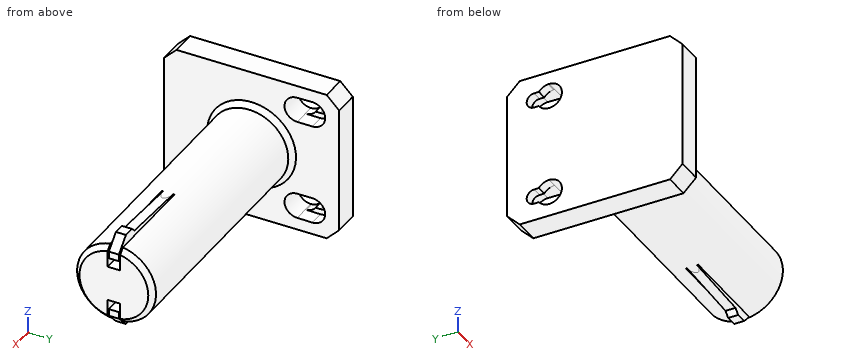
from build123d import *

# Parameters (mm, degrees)
SKETCH1_W            = 60.5
SKETCH1_H            = 70
BOSS_EXTRUDE1_DEPTH  = 10
SKETCH2_R            = 15.75
BOSS_EXTRUDE2_DEPTH  = 101.6
CUT_EXTRUDE1_DEPTH   = 40
SKETCH8_W            = 3.25
SKETCH8_H            = 5
CUT_EXTRUDE2_DEPTH   = 40
CHAMFER3_SIZE        = 2
BOSS_EXTRUDE9_DEPTH  = 4
BOSS_EXTRUDE10_DEPTH = 4
CHAMFER4_SIZE        = 5
CUT_EXTRUDE9_DEPTH   = 4
CHAMFER6_SIZE        = 2


with BuildPart() as part:
    # Sketch1 → Boss-Extrude1 (new body)
    with BuildSketch(Plane(origin=(0, 0, 0), x_dir=(0, 0, -1), z_dir=(1, 0, 0))):
        with Locations((0.23118778, -0.809157231)):
            Rectangle(SKETCH1_W, SKETCH1_H)
        with BuildLine():
            Line((-14.90655725, 23.440204594), (-14.924987971, 17.440316828))
            ThreePointArc((-14.924987971, 17.440316828), (-20.01881222, 12.34649258), (-25.112636468, 17.440316828))
            Line((-25.112636468, 17.440316828), (-25.204464795, 23.440204594))
            ThreePointArc((-25.204464795, 23.440204594), (-20.055511023, 28.589158366), (-14.90655725, 23.440204594))
        make_face(mode=Mode.SUBTRACT)
        with BuildLine():
            ThreePointArc((15.368932811, 23.440204594), (20.517886583, 28.589158366), (25.666840355, 23.440204594))
            Line((25.666840355, 23.440204594), (25.575012029, 17.440316828))
            ThreePointArc((25.575012029, 17.440316828), (20.48118778, 12.34649258), (15.387363532, 17.440316828))
            Line((15.387363532, 17.440316828), (15.368932811, 23.440204594))
        make_face(mode=Mode.SUBTRACT)
    extrude(amount=BOSS_EXTRUDE1_DEPTH)

    # Sketch2 → Boss-Extrude2 (add)
    with BuildSketch(Plane(origin=(10, 0, 0), x_dir=(0, 0, -1), z_dir=(1, 0, 0))):
        with Locations((0.23118778, -0.809157231)):
            Circle(SKETCH2_R)
    extrude(amount=BOSS_EXTRUDE2_DEPTH)

    # Sketch3 → Cut-Extrude1 (cut)
    with BuildSketch(Plane(origin=(111.6, 0, 0), x_dir=(0, 0, -1), z_dir=(1, 0, 0))):
        Polygon((-15.51881222, 1.190842769), (-10.51881222, 1.190842769), (-10.51881222, -2.809157231), (-15.51881222, -2.809157231), (-15.51881222, -3.309157231), (-10.01881222, -3.309157231), (-10.01881222, 1.690842769), (-15.51881222, 1.690842769), align=None)
        Polygon((15.98118778, -2.809157231), (15.98118778, -3.309157231), (10.48118778, -3.309157231), (10.48118778, 1.690842769), (15.98118778, 1.690842769), (15.98118778, 1.190842769), (10.98118778, 1.190842769), (10.98118778, -2.809157231), align=None)
    extrude(amount=-CUT_EXTRUDE1_DEPTH, mode=Mode.SUBTRACT)

    # Sketch8 → Cut-Extrude2 (cut)
    with BuildSketch(Plane(origin=(111.6, 0, 0), x_dir=(0, 0, -1), z_dir=(1, 0, 0))):
        with Locations((8.85618778, -0.809157231)):
            Rectangle(SKETCH8_W, SKETCH8_H)
        with Locations((-8.39381222, -0.809157231)):
            Rectangle(SKETCH8_W, SKETCH8_H)
    extrude(amount=-CUT_EXTRUDE2_DEPTH, mode=Mode.SUBTRACT)

    # Chamfer3
    chamfer3_edges = [part.edges().sort_by_distance(p)[0] for p in [
        (111.6, -16.559157231, -0.23118778),
        (111.6, 14.940842769, -0.23118778),
    ]]
    chamfer(chamfer3_edges, length=CHAMFER3_SIZE)

    # Sketch19 → Boss-Extrude9 (add)
    with BuildSketch(Plane.ZY):
        with BuildLine():
            Line((-25.666840355, 23.440204594), (-25.575012029, 17.440316828))
            ThreePointArc((-25.575012029, 17.440316828), (-25.569608823, 17.67487337), (-25.553410667, 17.908932306))
            ThreePointArc((-25.553410667, 17.908932306), (-24.917258091, 19.94397928), (-23.503874553, 21.540366846))
            Line((-23.503874553, 21.540366846), (-23.503874553, 23.440204594))
            ThreePointArc((-23.503874553, 23.440204594), (-20.517886583, 26.426192563), (-17.531898613, 23.440204594))
            Line((-17.531898613, 23.440204594), (-17.531898613, 21.593476936))
            ThreePointArc((-17.531898613, 21.593476936), (-15.9551406, 19.777396716), (-15.387363532, 17.440316828))
            Line((-15.387363532, 17.440316828), (-15.368932811, 23.440204594))
            ThreePointArc((-15.368932811, 23.440204594), (-20.517886583, 28.589158366), (-25.666840355, 23.440204594))
        make_face()
        with BuildLine():
            ThreePointArc((25.204464795, 23.440204594), (20.055511023, 28.589158366), (14.90655725, 23.440204594))
            Line((14.90655725, 23.440204594), (14.924987971, 17.440316828))
            ThreePointArc((14.924987971, 17.440316828), (15.49276504, 19.777396716), (17.069523053, 21.593476936))
            Line((17.069523053, 21.593476936), (17.069523053, 23.440204594))
            ThreePointArc((17.069523053, 23.440204594), (20.055511023, 26.426192563), (23.041498992, 23.440204594))
            Line((23.041498992, 23.440204594), (23.041498992, 21.540366846))
            ThreePointArc((23.041498992, 21.540366846), (24.454882531, 19.94397928), (25.091035106, 17.908932306))
            ThreePointArc((25.091035106, 17.908932306), (25.107233262, 17.67487337), (25.112636468, 17.440316828))
            Line((25.112636468, 17.440316828), (25.204464795, 23.440204594))
        make_face()
    extrude(amount=-BOSS_EXTRUDE9_DEPTH)

    # Sketch23 → Boss-Extrude10 (add)
    with BuildSketch(Plane(origin=(0, 1.190842769, 0), x_dir=(1, 0, 0), z_dir=(0, 1, 0))):
        Polygon((71.6, 15.78150932), (100.084633461, 17.181034874), (102.038578597, 19.029077367), (111.6, 19.029077367), (111.6, 15.78150932), align=None)
        Polygon((100.084633461, -16.718659314), (102.038578597, -18.566701807), (111.6, -18.566701807), (111.6, -15.31913376), (71.6, -15.31913376), align=None)
    extrude(amount=-BOSS_EXTRUDE10_DEPTH)

    # Chamfer4
    chamfer4_edges = [part.edges().sort_by_distance(p)[0] for p in [
        (5, -35.809157231, 30.01881222),
        (5, 34.190842769, 30.01881222),
        (5, 34.190842769, -30.48118778),
        (5, -35.809157231, -30.48118778),
    ]]
    chamfer(chamfer4_edges, length=CHAMFER4_SIZE)

    # Sketch28 → Cut-Extrude9 (cut)
    with BuildSketch(Plane(origin=(0, 1.190842769, 0), x_dir=(1, 0, 0), z_dir=(0, 1, 0))):
        Polygon((111.6, 13.752005063), (105.070544586, 20.392137095), (111.6, 20.392137095), align=None)
        Polygon((111.6, -19.929761535), (111.6, -13.289629503), (105.070544586, -19.929761535), align=None)
    extrude(amount=-CUT_EXTRUDE9_DEPTH, mode=Mode.SUBTRACT)

    # Chamfer6
    chamfer6_edges = [part.edges().sort_by_distance(p)[0] for p in [
        (10, -0.809157231, 15.51881222),
    ]]
    chamfer(chamfer6_edges, length=CHAMFER6_SIZE)


solid = part.part
The model under review builds one solid part; all positions refer to its coordinate system, in mm. Coordinates: 2 decimals unless noted, no trailing zeros. Loops run counter-clockwise (first coordinate to the right, second up) from the corner with the lowest first, then second, coordinate; pieces in that order, holes last.
(1) Consider section A-A, the plane y = 20. Give the boundary of the cut face in (x, z), plus the area to 3 significant figures.
Determined:
outline: (0, -30.48) - (10, -30.48) - (10, -25.61) - (4, -25.61) - (4, -24.89) - (0, -24.89) - close; (0, -16.08) - (4, -16.08) - (4, -15.38) - (10, -15.38) - (10, 14.92) - (4, 14.92) - (4, 15.61) - (0, 15.61) - close; (0, 24.42) - (4, 24.42) - (4, 25.15) - (10, 25.15) - (10, 30.02) - (0, 30.02) - close
area: 412 mm2
(2) Insertion check: P1, Ø7, axis at x = 99, z = -13.5, coming from the -Y side; P2, Ø8, axis at x = 25.5, z = 11.5, coming from the -Y side; P3, Ø3, axis at y = 20.5, z = 20.5, coming from the +X side; P4, Ø11.5, axis at y = 21, z = -22, coming from the +X side. Each pin has a flat end and moves straight along its axis. Give the tip position at first contact, or say it passes through.
Determined:
P1: stops at y = -13.16
P2: stops at y = -14.53
P3: passes through
P4: stops at x = 10
(3) Consider section B-B, the plane x = 81. Give the boundary of the cut face in (y, z).
Determined:
outline: (-3.31, -15.78) - (-3.31, -7.23) - (1.69, -7.23) - (1.69, -15.78) arc R15.75 ccw to (1.69, 15.32) - (1.69, 6.77) - (-3.31, 6.77) - (-3.31, 15.32) arc R15.75 ccw to start; (-2.81, -16.24) - (1.19, -16.24) - (1.19, -10.98) - (-2.81, -10.98) - close; (-2.81, 10.52) - (1.19, 10.52) - (1.19, 15.78) - (-2.81, 15.78) - close
(4) Consider section C-C, the plane z = 21. Give the boundary of the cut face in (x, y), plus the area to 3 significant figures.
Determined:
outline: (0, -35.81) - (10, -35.81) - (10, 12.44) - (0, 12.44) - close; (0, 26.27) - (4, 26.27) - (4, 28.5) - (10, 28.5) - (10, 34.19) - (0, 34.19) - close
area: 548 mm2
(5) Wall thickness on L1, parallel to X at y = 22, z = -25; L2, parallel to X at y = -29.5, z = 27.5; L3, parallel to Z at x = 41.5, y = -0.5: over which ranges is each line inside the solid? List them lowest first.
Determined:
L1: x = 0 to 4
L2: x = 0 to 10
L3: z = -15.98 to 15.52
(6) Consider section D-D, the plane y = -23. Give the boundary of the cut face in (x, z), plus the area to 3 significant figures.
Determined:
outline: (0, -30.48) - (10, -30.48) - (10, 30.02) - (0, 30.02) - close
area: 605 mm2
